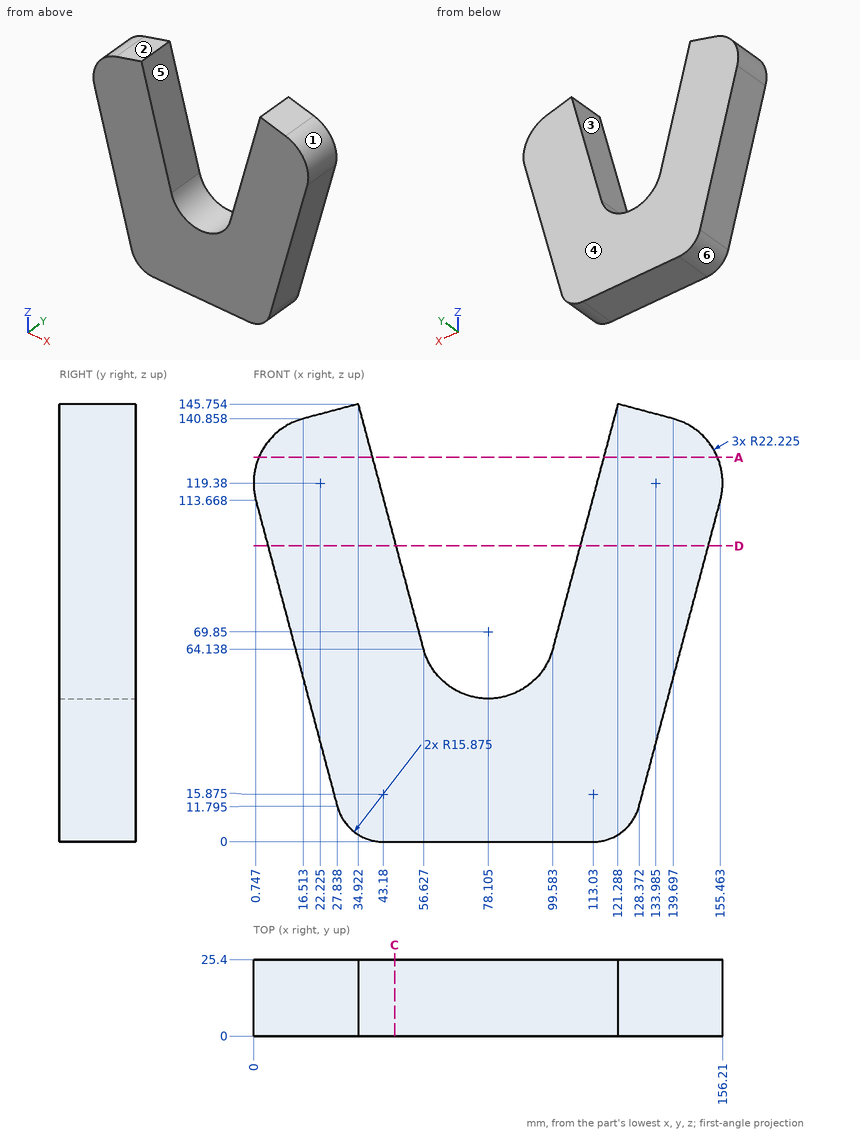
Here's the drawing with two shaded views (mm, measured from the low corner). I have some questions. A direction names the side the tool comes from. Round coordinates to 2 decimals unless told otherwise and drop trailing zeros. Loops run counter-clockwise (first coordinate to the right, second up) from the corner with the lowest first, then second, coordinate; pieces in that order, holes last. Notation, with made-up numbers: M 56,-19.5 L 81,-19.5 A24 ccw 81,-1.5 Z; hole C 85.25,25 d3. An arc over 180 degrees is marked long. Answer as a JSON object with one key per item and string values. Group by question number.
Q1. Please list where these lines run through material, in increasing order: L1, parallel to X at y = 9, z = 76 (1 decimal); L2, parallel to X at y = 12.5, z = 69.5; L3, parallel to Z at x = 30.5, y = 9 (1 decimal).
Q2. Will these pins go through, and if not, where does the flat tip stop? pin 1 (5 mm diameter, centred on x = 34, y = 18.5, fed in from -Z) (1 decimal); pin 2 (5 mm diameter, centred on y = 14, z = 126, fed in from +X) (1 decimal); pin 3 (4 mm diameter, centred on x = 28, y = 8, fed in from +Z) (1 decimal); pin 4 (12 mm diameter, centred on x = 113, z = 78.5, fed in from -Y).
Q3. Imagine slicing it at D-D, the plane z = 98.5. Please give me the cut outline in (x, y).
Q4. Imagine slicing it at C-C, the plane x = 47. Please give me the cut outline in (y, z).
Q5. Imagine slicing it at A-A, the plane z = 128. Please give me the cut outline in (x, y), then the cut area to 3 significant figures.
Q6. We'd pull the mould along X, two halves only. Please class the marked faces 1, 2, 3 and 4: +X half, -X half, draft (parallel to the pull), parting line (faces both ways), or undercut.
Q7. On a 3-axis mill with a long thin cutter (end or side, diameter ignored), from which of +Z, -Z, +X, -X, +Y, -Y can I reach the whole of each face in a straight line? I mean the marked faces 5 and 6. Say none if no direction works.
Findings:
{
 "1": {"L1": "x = 10.8 to 53.5, 102.7 to 145.4", "L2": "x = 12.49 to 55.2, 101.01 to 143.72", "L3": "z = 6.3 to 144.6"},
 "2": {"pin 1": "stops at z = 1.5", "pin 2": "stops at x = 155.8", "pin 3": "stops at z = 144.4", "pin 4": "stops at y = 0"},
 "3": {"outline": "M 4.78,0 L 47.49,0 L 47.49,25.4 L 4.78,25.4 Z; M 108.72,0 L 151.43,0 L 151.43,25.4 L 108.72,25.4 Z"},
 "4": {"outline": "M 0,0 L 25.4,0 L 25.4,100.34 L 0,100.34 Z"},
 "5": {"outline": "M 1.74,0 L 39.64,0 L 39.64,25.4 L 1.74,25.4 Z; M 116.57,0 L 154.47,0 L 154.47,25.4 L 116.57,25.4 Z", "area": "1,930 mm2"},
 "6": {"face 1": "+X half", "face 2": "-X half", "face 3": "undercut", "face 4": "draft"},
 "7": {"face 5": "+Z, +Y, -Y", "face 6": "-Z, -X, +Y, -Y"}
}
